Input: dimensioned drawing with shaded views. Units: mm. Origin: part minimum x, y, z. A direction names the side the tool comes from. Give positions to 0.01 mm unless a question says otherwise; leave off trailing zeros. Write each loop counter-clockwise with the first axis right and the second up, starting at its lowest first coordinate (ties: lowest second). Pieces come first, ordered by that corner, then holes.
Q1. Section A-A (y = 5.5). Return the cut outline in (x, z), plus the area to 3 significant figures.
Q2. Line query: line 1 (Z direction, x = 1.25, y = 12.75); line 2 (Y direction, x = 11, z = 21). Output: solid intervals per line, ascending.
Q3. Section C-C (x = 4.25). Return the cut outline in (y, z).
Q4. Pin query (flat end, axial travel): pin 1 Ø7.5 at (x, z) = (7.5, 15.5) entering from +Y. Return the tip coordinate at first contact, or that it passes through.
Q5. Section B-B (z = 29.5). Return the cut outline in (x, y).
Q6. Mould query, pull axis X, two halves, no side actions, for the marked faces 3, 4 and 5. Classes: +X half, -X half, draft (parallel to the pull), parting line (faces both ways), or undercut.
Q7. Reachability of the marked faces 1 and 2 from +Z, -Z, +X, -X, +Y, -Y: full face, straight path, thin tool, end or side. Return the list, or none.
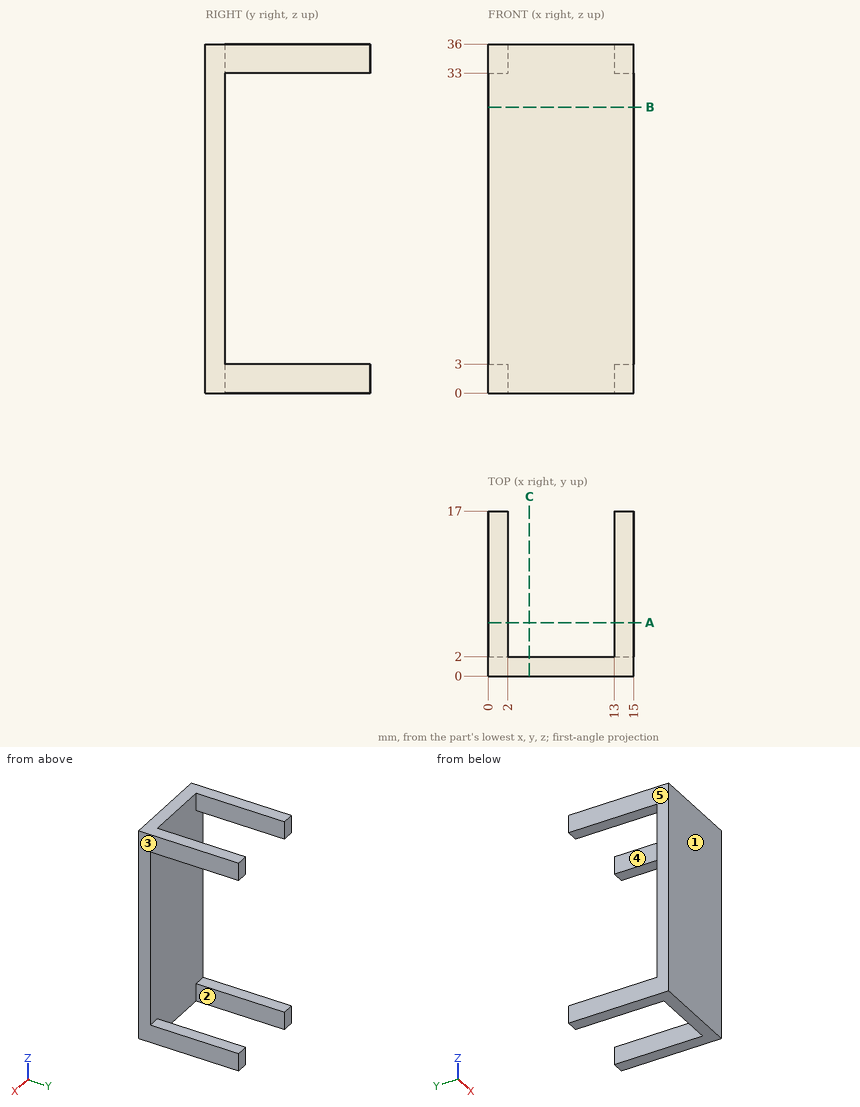
Computed:
1. outline: (0, 0) - (2, 0) - (2, 3) - (0, 3) - close; (0, 33) - (2, 33) - (2, 36) - (0, 36) - close; (13, 0) - (15, 0) - (15, 3) - (13, 3) - close; (13, 33) - (15, 33) - (15, 36) - (13, 36) - close
1. area: 24.0 mm2
2. line 1: z = 0 to 3, 33 to 36
2. line 2: y = 0 to 2
3. outline: (0, 0) - (2, 0) - (2, 36) - (0, 36) - close
4. pin 1: stops at y = 2
5. outline: (0, 0) - (15, 0) - (15, 2) - (0, 2) - close
6. face 3: +X half
6. face 4: undercut
6. face 5: -X half
7. face 1: +Z, -Z, +X, -X, -Y
7. face 2: +Z, -Z, +Y
